from build123d import *

# Parameters (mm, degrees)
F2_R     = 25.25
F3_DEPTH = 4
F4_R     = 24
F5_DEPTH = 16
F6_R     = 29.5
F6_R_2   = 25.25
F7_DEPTH = 2.5
F9_D     = 2
F9_DEPTH = 5
F9_TIP   = 0.600860619


with BuildPart() as f1:
    # F0 (on Right) → F1 (revolve)
    with BuildSketch(Plane.YZ):
        Polygon((0, 36), (0, 0), (20, 0), (20, 36), (16, 36), (16, 30), (12, 30), (6, 36), align=None)
    revolve(axis=Axis((0, 10, 0), (0, -1, 0)))

    # F2 (on face) → F3 (cut)
    with BuildSketch(Plane.XZ):
        Circle(F2_R)
    extrude(amount=-F3_DEPTH, mode=Mode.SUBTRACT)

    # F4 (on face) → F5 (cut, through all)
    with BuildSketch(Plane.XZ.offset(-4)):
        Circle(F4_R)
    extrude(amount=-F5_DEPTH, mode=Mode.SUBTRACT)

    # F6 (on face) → F7 (cut)
    with BuildSketch(Plane.XZ):
        Circle(F6_R)
        Circle(F6_R_2, mode=Mode.SUBTRACT)
    extrude(amount=-F7_DEPTH, mode=Mode.SUBTRACT)

    # F9
    with Locations(Plane.XZ.offset(-2.5)):
        with Locations((0, 26.75), (23.1661795512, -13.375), (-23.1661795512, -13.375)):
            Hole(F9_D / 2, depth=F9_DEPTH)
            with Locations((0, 0, -(F9_DEPTH + F9_TIP / 2))):  # 118° drill point
                Cone(0, F9_D / 2, F9_TIP, mode=Mode.SUBTRACT)


solid = f1.part
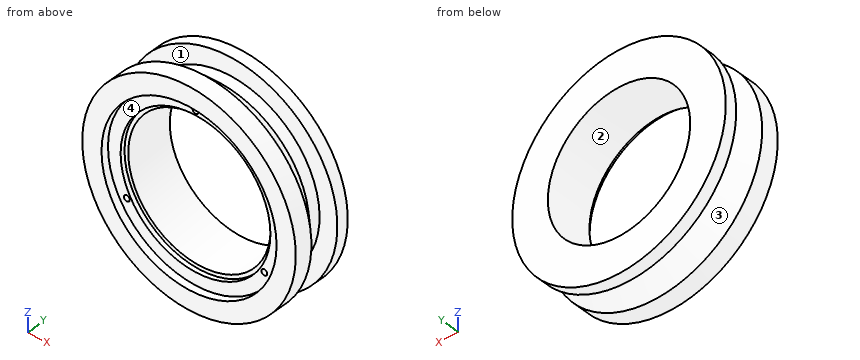
Input: part model. Units: mm. Frame: model coordinates. Face numbers are marked on the shaded views. Give positions to 0.01 mm unless a question says otherwise; leave off trailing zeros. Write each loop counter-clockwise with the first axis right and the second up, starting at its lowest first coordinate (ties: lowest second). Pieces come first, ordered by that corner, then holes.
Q1. Section A-A, the plane z = 0. Output: boundary loops of the cut face in (x, y), plus the area to 3 significant figures.
Q2. First-contact query: P1, Ø8, axis at y = 12.5, z = -7, coming from the +X side; P2, Ø1.6, axis at x = -23.17, z = -13.38, coming from the -Y side; P3, Ø3, axis at x = -4.5, y = 5, coming from the +Z side. Flat tips, straight axial feed; report the tip coordinate or a pass-through.
Q3. Material intervals for probe 1 along Z at (x, y) = (0, 12); probe 2 along Z at (x, y) = (0, 5.2); probe 3 along X at (y, z) = (6, 0.5), sorted ascending.
Q4. Section B-B, the plane y = 13.5. Output: boundary loops of the cut face in (x, z), plus the area to 3 significant figures.
Q5. Pull-direction query (X, two-part tool) for the marked faces 1, 2, 3 and 4; classes: pulls with the +X half, pulls with the -X half, needs draft (parallel to the pull), parting line crosses it, or undercut.
Filled in:
1. outline: (-36, 0) - (-29.5, 0) - (-29.5, 2.5) - (-25.25, 2.5) - (-25.25, 4) - (-24, 4) - (-24, 20) - (-36, 20) - (-36, 16) - (-30, 16) - (-30, 12) - (-36, 6) - close; (24, 4) - (25.25, 4) - (25.25, 2.5) - (29.5, 2.5) - (29.5, 0) - (36, 0) - (36, 6) - (30, 12) - (30, 16) - (36, 16) - (36, 20) - (24, 20) - close
1. area: 365 mm2
2. P1: stops at x = 35.64
2. P2: stops at y = 7.62
2. P3: stops at z = 35.87
3. probe 1: z = -30 to -24, 24 to 30
3. probe 2: z = -36 to -24, 24 to 25.75, 27.75 to 36
3. probe 3: x = -36 to -23.99, 23.99 to 36
4. outline: circle Ø60 at (0, 0); hole circle Ø48 at (0, 0)
4. area: 1,020 mm2
5. face 1: needs draft
5. face 2: undercut
5. face 3: parting line crosses it
5. face 4: undercut
